```python
from build123d import *

# Parameters (mm, degrees)
SKETCH1_R           = 3.302
BOSS_EXTRUDE1_DEPTH = 1.5875


with BuildPart() as part:
    # Sketch1 → Boss-Extrude1 (new body)
    with BuildSketch(Plane.XY):
        Polygon((29.845, -3.175), (31.4325, -3.175), (31.4325, 3.175), (29.845, 3.175), (29.845, 6.35), (-29.845, 6.35), (-29.845, 3.175), (-31.4325, 3.175), (-31.4325, -3.175), (-29.845, -3.175), (-29.845, -6.35), (29.845, -6.35), align=None)
        with Locations((-22.86, 0)):
            Circle(SKETCH1_R, mode=Mode.SUBTRACT)
        with Locations((22.86, 0)):
            Circle(SKETCH1_R, mode=Mode.SUBTRACT)
    extrude(amount=-BOSS_EXTRUDE1_DEPTH)


solid = part.part
```
Verification items for the finished model (mm, model axes). A direction names the side the tool comes from. Give positions to 0.01 mm unless a question says otherwise; leave off trailing zeros. Write each loop counter-clockwise with the first axis right and the second up, starting at its lowest first coordinate (ties: lowest second). Pieces come first, ordered by that corner, then holes. Notation, with made-up numbers: M 71,-14 L 128,-14 A17 cw 128,-8 Z; hole C -11.75,79 d4. An arc over 180 degrees is marked long. One line per question, with ' | ' between items.
1) Gauge pin test, flat ends, axial feed: pin 1 Ø0.8 at (y, z) = (4, -1) entering from +X (3 decimals); pin 2 Ø0.5 at (y, z) = (-5.5, -1) entering from -X (3 decimals); pin 3 Ø0.8 at (x, z) = (-30.5, -1) entering from +Y (3 decimals). Record the tip position at first contact, or that the pin passes through.
Result:
pin 1: stops at x = 29.845 | pin 2: stops at x = -29.845 | pin 3: stops at y = 3.175
2) Section check B-B on z = -1. State how many separate pieces and enclosed holes the cut face has, plus the area to 3 significant figures.
Result:
separate pieces: 1 | enclosed holes: 2 | area: 710 mm2
3) Set-up check for faces 4 (the flat face through (-29.845, 5, -1)), 5 (the flat face through (31, -3.175, -1)), 6 (the flat face through (29.845, 5, -1)), 7 (the flat face through (-31, -3.175, -1)): record each of +Z, -Z, +X, -X, +Y, -Y from which the full face is reachable in a straight line by a thin tool's end or side.
Result:
face 4: +Z, -Z, -X, +Y | face 5: +Z, -Z, +X, -Y | face 6: +Z, -Z, +X, +Y | face 7: +Z, -Z, -X, -Y
4) Section check D-D on y = -4.5. Enter the section's corners in (x, z) (1 decimal).
Result:
outline: M -29.8,-1.6 L 29.8,-1.6 L 29.8,0 L -29.8,0 Z
5) Section check A-A on y = 0. Enter the section's corners in (x, z).
Result:
outline: M -31.43,-1.59 L -26.16,-1.59 L -26.16,0 L -31.43,0 Z; M -19.56,-1.59 L 19.56,-1.59 L 19.56,0 L -19.56,0 Z; M 26.16,-1.59 L 31.43,-1.59 L 31.43,0 L 26.16,0 Z
6) Section check C-C on x = -22.5. Enter the section's corners in (y, z).
Result:
outline: M -6.35,-1.59 L -3.28,-1.59 L -3.28,0 L -6.35,0 Z; M 3.28,-1.59 L 6.35,-1.59 L 6.35,0 L 3.28,0 Z
7) Mould release check, pull along X, two halves, no side actions. Record for faces 1 (the cylindrical face through (26.01, 0.99, -0.78)), 2 (the flat face through (0, 0, -1.588)), 3 (the flat face through (29.845, -5, -1)): released by +X, released by -X, zero draft, split by the parting line, or undercut.
Result:
face 1: undercut | face 2: zero draft | face 3: released by +X
8) Thickness scan on line 1 along Y through (x, z) = (22.86, -0.45); line 2 along X through (y, z) = (-1.75, -0.75); line 3 along X through (y, z) = (-2.75, -0.55). Record the ranges inside material, lowest first. Write a range as [from, to].
Result:
line 1: y = [-6.35, -3.3], [3.3, 6.35] | line 2: x = [-31.43, -25.66], [-20.06, 20.06], [25.66, 31.43] | line 3: x = [-31.43, -24.69], [-21.03, 21.03], [24.69, 31.43]
